```python
from build123d import *

# Parameters (mm, degrees)
SKETCH1_W                                        = 76.2
SKETCH1_H                                        = 125
BOSS_EXTRUDE1_DEPTH                              = 7.9375
CBORE_FOR_1_4_BUTTON_HEAD_CAP_SCREW1_D           = 6.5278
CBORE_FOR_1_4_BUTTON_HEAD_CAP_SCREW1_DEPTH       = 7.9375
CBORE_FOR_1_4_BUTTON_HEAD_CAP_SCREW1_CBORE_D     = 11.90752
CBORE_FOR_1_4_BUTTON_HEAD_CAP_SCREW1_CBORE_DEPTH = 3.3528
M3X0_5_TAPPED_HOLE1_D                            = 2.5
M3X0_5_TAPPED_HOLE1_DEPTH                        = 7.9375
F_10_32_TAPPED_HOLE1_D                           = 4.0386
F_10_32_TAPPED_HOLE1_DEPTH                       = 10.16
F_10_32_TAPPED_HOLE1_TIP                         = 1.213317848
F_10_32_TAPPED_HOLE2_D                           = 4.0386
F_10_32_TAPPED_HOLE2_DEPTH                       = 10.16
F_10_32_TAPPED_HOLE2_TIP                         = 1.213317848
CUT_EXTRUDE1_DEPTH                               = 4.7625


with BuildPart() as part:
    # Sketch1 → Boss-Extrude1 (new body)
    with BuildSketch(Plane.XY):
        Rectangle(SKETCH1_W, SKETCH1_H)
    extrude(amount=BOSS_EXTRUDE1_DEPTH)

    # CBORE for 1/4 Button Head Cap Screw1
    with Locations(Plane.XY.offset(7.9375)):
        with Locations((-19.05, 38.1), (19.05, 38.1), (19.05, -38.1), (-19.05, -38.1)):
            CounterBoreHole(CBORE_FOR_1_4_BUTTON_HEAD_CAP_SCREW1_D / 2, CBORE_FOR_1_4_BUTTON_HEAD_CAP_SCREW1_CBORE_D / 2, CBORE_FOR_1_4_BUTTON_HEAD_CAP_SCREW1_CBORE_DEPTH, depth=CBORE_FOR_1_4_BUTTON_HEAD_CAP_SCREW1_DEPTH)

    # M3x0.5 Tapped Hole1
    with Locations(Plane.XY.offset(7.9375)):
        with Locations((-22.225, 50), (-22.225, 25), (-22.225, 0), (-22.225, -25), (-22.225, -50), (22.225, -50), (22.225, -25), (22.225, 0), (22.225, 25), (22.225, 50)):
            Hole(M3X0_5_TAPPED_HOLE1_D / 2, depth=M3X0_5_TAPPED_HOLE1_DEPTH)

    # #10-32 Tapped Hole1
    with Locations(Plane(origin=(0, 62.5, 0), x_dir=(1, 0, 0), z_dir=(0, 1, 0))):
        with Locations((-19.05, -3.96875), (19.05, -3.96875)):
            Hole(F_10_32_TAPPED_HOLE1_D / 2, depth=F_10_32_TAPPED_HOLE1_DEPTH)
            with Locations((0, 0, -(F_10_32_TAPPED_HOLE1_DEPTH + F_10_32_TAPPED_HOLE1_TIP / 2))):  # 118° drill point
                Cone(0, F_10_32_TAPPED_HOLE1_D / 2, F_10_32_TAPPED_HOLE1_TIP, mode=Mode.SUBTRACT)

    # #10-32 Tapped Hole2
    with Locations(Plane(origin=(0, -62.5, 0), x_dir=(-1, 0, 0), z_dir=(0, -1, 0))):
        with Locations((19.05, -3.96875), (-19.05, -3.96875)):
            Hole(F_10_32_TAPPED_HOLE2_D / 2, depth=F_10_32_TAPPED_HOLE2_DEPTH)
            with Locations((0, 0, -(F_10_32_TAPPED_HOLE2_DEPTH + F_10_32_TAPPED_HOLE2_TIP / 2))):  # 118° drill point
                Cone(0, F_10_32_TAPPED_HOLE2_D / 2, F_10_32_TAPPED_HOLE2_TIP, mode=Mode.SUBTRACT)

    # Sketch10 → Cut-Extrude1 (cut)
    with BuildSketch(Plane(origin=(0, 0, 0), x_dir=(-1, 0, 0), z_dir=(0, 0, -1))):
        with BuildLine():
            Line((7.9375, -60.325), (-7.9375, -60.325))
            ThreePointArc((-7.9375, -60.325), (-11.305096045, -58.930096045), (-12.7, -55.5625))
            Line((-12.7, -55.5625), (-12.7, 55.5625))
            ThreePointArc((-12.7, 55.5625), (-11.305096045, 58.930096045), (-7.9375, 60.325))
            Line((-7.9375, 60.325), (7.9375, 60.325))
            ThreePointArc((7.9375, 60.325), (11.305096045, 58.930096045), (12.7, 55.5625))
            Line((12.7, 55.5625), (12.7, -55.5625))
            ThreePointArc((12.7, -55.5625), (11.305096045, -58.930096045), (7.9375, -60.325))
        make_face()
        with BuildLine():
            Line((-25.4, 55.5625), (-25.4, -55.5625))
            ThreePointArc((-25.4, -55.5625), (-30.1625, -60.325), (-34.925, -55.5625))
            Line((-34.925, -55.5625), (-34.925, 55.5625))
            ThreePointArc((-34.925, 55.5625), (-30.1625, 60.325), (-25.4, 55.5625))
        make_face()
        with BuildLine():
            Line((34.925, 55.5625), (34.925, -55.5625))
            ThreePointArc((34.925, -55.5625), (30.1625, -60.325), (25.4, -55.5625))
            Line((25.4, -55.5625), (25.4, 55.5625))
            ThreePointArc((25.4, 55.5625), (30.1625, 60.325), (34.925, 55.5625))
        make_face()
    extrude(amount=-CUT_EXTRUDE1_DEPTH, mode=Mode.SUBTRACT)


solid = part.part
```
Check sheet for the modelled part. Datum: model origin and axes. Units: mm. A direction names the side the tool comes from. Round coordinates to 2 decimals unless told otherwise and drop trailing zeros. Order: outer loops, then holes, each group sorted by start corner. A loop starts at its lowest first (then second) coordinate and runs counter-clockwise, first axis right, second up. Notation, with made-up numbers: (-8, 35) - (25, 35) arc R19 ccw to (25, 41) - close; hole circle Ø9 at (0, -12.5). An arc over 180 degrees is marked (long way). Write item = value, one per line.
Q1. Tool access check on faces 5 (the face through (-25.4, -1, 2)), 6 (the face through (19.475, 41.336, 2.26)), 7 (the face through (-19.825, 44.003, 6.285)). Record the directions out of +Z, -Z, +X, -X, +Y, -Y that give a thin tool (end or side, any length) a straight path to the whole face; none if there is none.
Computed:
face_5 = -Z
face_6 = +Z, -Z
face_7 = +Z
Q2. Section check A-A (y = 25). Record the boundary of the cut face in (x, z) (1 decimal).
Computed:
outline = (-38.1, 0) - (-34.9, 0) - (-34.9, 4.8) - (-25.4, 4.8) - (-25.4, 0) - (-23.5, 0) - (-23.5, 7.9) - (-38.1, 7.9) - close; (-21, 0) - (-12.7, 0) - (-12.7, 4.8) - (12.7, 4.8) - (12.7, 0) - (21, 0) - (21, 7.9) - (-21, 7.9) - close; (23.5, 0) - (25.4, 0) - (25.4, 4.8) - (34.9, 4.8) - (34.9, 0) - (38.1, 0) - (38.1, 7.9) - (23.5, 7.9) - close
Q3. Go/stop test with flat-tipped pins: pin 1 (1.5 mm diameter, centred on x = -22.225, y = -50, fed in from +Z); pin 2 (3 mm diameter, centred on x = 29.5, y = -32, fed in from -Z). Record where each tip stops, or that it passes through.
Computed:
pin_1 = through
pin_2 = 4.76
Q4. Section check D-D (y = -38.1). State how many separate pieces and enclosed holes the cut face has, and give its area (3 significant figures).
Computed:
separate_pieces = 3
enclosed_holes = 0
area = 253 mm^2
Q5. Thickness scan on line 1 along X through (y, z) = (16, 0.75) (3 decimals); line 2 along X through (y, z) = (40, 7.5); line 3 along X through (y, z) = (-57, 5.25). Record the ranges inside material, lowest first.
Computed:
line_1 = -38.1 to -34.925, -25.4 to -12.7, 12.7 to 25.4, 34.925 to 38.1
line_2 = -38.1 to -24.69, -13.41 to 13.41, 24.69 to 38.1
line_3 = -38.1 to -20.61, -17.49 to 17.49, 20.61 to 38.1
Q6. Section check B-B (y = -19). Record the boundary of the cut face in (x, z) (1 decimal), and give its area (3 significant figures).
Computed:
outline = (-38.1, 0) - (-34.9, 0) - (-34.9, 4.8) - (-25.4, 4.8) - (-25.4, 0) - (-12.7, 0) - (-12.7, 4.8) - (12.7, 4.8) - (12.7, 0) - (25.4, 0) - (25.4, 4.8) - (34.9, 4.8) - (34.9, 0) - (38.1, 0) - (38.1, 7.9) - (-38.1, 7.9) - close
area = 393 mm^2
Q7. Draft check along Y on faces 1 (the face through (22, -41, 4.585)), 2 (the face through (18.716, -51.337, 3.863)), 3 (the face through (14, 10, 0)), 4 (the face through (-12.7, 1, 2)). Enter one of: pulls with the +Y half, pulls with the -Y half, needs draft (parallel to the pull), parting line crosses it, or undercut.
Computed:
face_1 = undercut
face_2 = pulls with the -Y half
face_3 = needs draft
face_4 = undercut
Q8. Section check C-C (x = -1). Record the boundary of the cut face in (y, z) (1 decimal), and give its area (3 significant figures).
Computed:
outline = (-62.5, 0) - (-60.3, 0) - (-60.3, 4.8) - (60.3, 4.8) - (60.3, 0) - (62.5, 0) - (62.5, 7.9) - (-62.5, 7.9) - close
area = 418 mm^2
